from build123d import *

# Parameters (mm, degrees)
SKETCH_1_R      = 35
EXTRUDE_1_DEPTH = 10
SKETCH_2_R      = 25
EXTRUDE_2_DEPTH = 136
SKETCH_3_R      = 18
EXTRUDE_3_DEPTH = 7
SKETCH_4_R      = 25
EXTRUDE_4_DEPTH = 12
CHAMFER_1_SIZE  = 2
CHAMFER_1_SIZE2 = 1.154700538
FILLET_1_R      = 1


with BuildPart() as part:
    # 草图1 → 凸台-拉伸1 (new body)
    with BuildSketch(Plane.XY):
        Circle(SKETCH_1_R)
    extrude(amount=EXTRUDE_1_DEPTH)

    # 草图2 → 凸台-拉伸2 (add)
    with BuildSketch(Plane.XY.offset(10)):
        Circle(SKETCH_2_R)
    extrude(amount=EXTRUDE_2_DEPTH)

    # 草图3 → 凸台-拉伸3 (add)
    with BuildSketch(Plane.XY.offset(146)):
        Circle(SKETCH_3_R)
    extrude(amount=EXTRUDE_3_DEPTH)

    # 草图4 → 凸台-拉伸4 (add)
    with BuildSketch(Plane.XY.offset(153)):
        Circle(SKETCH_4_R)
    extrude(amount=EXTRUDE_4_DEPTH)

    # 倒角1
    chamfer_1_edges = [part.edges().sort_by_distance(p)[0] for p in [
        (-25, 0, 165),
    ]]
    chamfer_1_side = [part.faces().sort_by_distance(p)[0] for p in [
        (-25, 0, 159),
    ]]
    chamfer(chamfer_1_edges, length=CHAMFER_1_SIZE, length2=CHAMFER_1_SIZE2, reference=chamfer_1_side[0])

    # 圆角1
    fillet_1_edges = [part.edges().sort_by_distance(p)[0] for p in [
        (-25, 0, 10),
    ]]
    fillet(fillet_1_edges, radius=FILLET_1_R)


solid = part.part
Design review of the part built by this model. Coordinates are the model's own, in mm. A direction names the side the tool comes from. Coordinates: 2 decimals unless noted, no trailing zeros. Write each loop counter-clockwise with the first axis right and the second up, starting at its lowest first coordinate (ties: lowest second). Pieces come first, ordered by that corner, then holes. Notation, with made-up numbers: (30, 52) - (68, 52) arc R8 cw to (68, 56) - close; hole circle Ø8 at (-12, -20). An arc over 180 degrees is marked (long way). Use one line per item in the form item = value.
Q1. Consider section A-A (x = 0). Write out the cut boundary in (y, z).
Taken from the geometry:
outline = (-35, 0) - (35, 0) - (35, 10) - (26, 10) arc R1 cw to (25, 11) - (25, 146) - (18, 146) - (18, 153) - (25, 153) - (25, 163) - (23.85, 165) - (-23.85, 165) - (-25, 163) - (-25, 153) - (-18, 153) - (-18, 146) - (-25, 146) - (-25, 11) arc R1 cw to (-26, 10) - (-35, 10) - close
Q2. The part is to be moulded in two halves that separate along Z. For faces 4 (the flat face through (-26.1, -2.4, 10)), 5 (the flat face through (11, -16, 153)), 6 (the cylindrical face through (-28, -21, 5)), 7 (the cylindrical face through (-2.343, 17.847, 149.451)), say which applies: +Z half, -Z half, draft (parallel to the pull), parting line (faces both ways), or undercut.
Taken from the geometry:
face_4 = +Z half
face_5 = undercut
face_6 = draft
face_7 = undercut
Q3. For probe 1 along Z at (x, y) = (-10, 18); probe 2 along Z at (x, y) = (14, -24.5); probe 3 along Y at (x, z) = (-1, 58), list the stretches that pass through material, from the lowest coordinate up.
Taken from the geometry:
probe_1 = 0 to 146, 153 to 165
probe_2 = 0 to 10
probe_3 = -24.98 to 24.98
Q4. Insertion check: pin 1 Ø10 at (x, z) = (13, 110) entering from +Y; pin 2 Ø6 at (y, z) = (9.5, 85) entering from -X; pin 3 Ø12 at (x, z) = (-24.5, 133) entering from +Y. Each pin has a flat end and moves straight along its axis. Give the tip position at first contact, or say it passes through.
Taken from the geometry:
pin_1 = 23.69
pin_2 = -24.14
pin_3 = 16.82
Q5. Consider section D-D (y = 29). Write out the cut boundary in (x, z), plus the area to 3 significant figures.
Taken from the geometry:
outline = (-19.6, 0) - (19.6, 0) - (19.6, 10) - (-19.6, 10) - close
area = 392 mm^2
Q6. Machinability: for faces 1 (the flat face through (0, 0, 0)), 2 (the flat face through (11, -16, 146)), 3 (the cylindrical face through (23.846, 7.509, 77.555)), which of the approach directions +Z, -Z, +X, -X, +Y, -Y give a long, thin tool a straight path to every point of the face, cutting with its end or side? Answer none if there is none.
Taken from the geometry:
face_1 = -Z, +X, -X, +Y, -Y
face_2 = none
face_3 = +Z
Q7. Consider section C-C (z = 58.5). Write out the cut boundary in (x, y), plus the area to 3 significant figures.
Taken from the geometry:
outline = circle Ø50 at (0, 0)
area = 1,960 mm^2
